from build123d import *

# Parameters (mm, degrees)
SKETCH_1_R          = 2.3
EXTRUDE_1_DEPTH     = 12
SKETCH_2_R          = 5.05
CUT_EXTRUDE_1_DEPTH = 3
CUT_EXTRUDE_START   = -3
SKETCH_3_R          = 5.05
CUT_EXTRUDE_2_DEPTH = 3
SKETCH_4_R          = 4
CUT_EXTRUDE_3_DEPTH = 15
CUT_EXTRUDE_4_DEPTH = 15
CHAMFER_1_SIZE      = 3
EXTRUDE_2_DEPTH     = 12
SKETCH_8_R          = 3
CUT_EXTRUDE_5_DEPTH = 12
CHAMFER_2_SIZE      = 3
SKETCH_9_R          = 2.3
EXTRUDE_4_DEPTH     = 4
FILLET_1_R          = 0.5
CUT_EXTRUDE_6_DEPTH = 22
SKETCH_11_R         = 4.05
CUT_EXTRUDE_7_DEPTH = 3
FILLET_2_R          = 0.5


with BuildPart() as part:
    # 草图1 → 凸台-拉伸1 (new body)
    with BuildSketch(Plane.XY):
        Polygon((-3.615367776, 90), (-7.5, -40), (-7.5, -80), (7.5, -80), (7.5, -40), (3.615367776, 90), align=None)
        with Locations((0, -74)):
            Circle(SKETCH_1_R, mode=Mode.SUBTRACT)
    extrude(amount=EXTRUDE_1_DEPTH)

    # 草图2 → 切除-拉伸1 (cut)
    with BuildSketch(Plane.XY.offset(12)):
        with Locations((0, -45)):
            Circle(SKETCH_2_R)
    extrude(amount=-CUT_EXTRUDE_1_DEPTH, mode=Mode.SUBTRACT)

    # 草图3 → 切除-拉伸2 (cut)
    with BuildSketch(Plane(origin=(0, 0, 0), x_dir=(-1, 0, 0), z_dir=(0, 0, -1)).offset(CUT_EXTRUDE_START)):
        with Locations(Location((0, -45, 0), (0, 0, 180))):
            Circle(SKETCH_3_R)
    extrude(amount=CUT_EXTRUDE_2_DEPTH, mode=Mode.SUBTRACT)

    # 草图4 → 切除-拉伸3 (cut)
    with BuildSketch(Plane.XY.offset(9)):
        with Locations((0, -45)):
            Circle(SKETCH_4_R)
    extrude(amount=-CUT_EXTRUDE_3_DEPTH, mode=Mode.SUBTRACT)

    # 草图6 → 切除-拉伸4 (cut)
    with BuildSketch(Plane.XY.offset(12)):
        Polygon((4.888073513, -27.298220102), (4.403458128, -9.298220102), (-4.403458128, -9.298220102), (-4.888073513, -27.298220102), align=None)
        Polygon((-3.86499659, 10.701779898), (3.86499659, 10.701779898), (4.349611974, -7.298220102), (-4.349611974, -7.298220102), align=None)
        Polygon((-2.734227359, 52.701779898), (2.734227359, 52.701779898), (2.249611974, 70.701779898), (-2.249611974, 70.701779898), align=None)
        Polygon((-3.272688897, 32.701779898), (3.272688897, 32.701779898), (2.788073513, 50.701779898), (-2.788073513, 50.701779898), align=None)
        Polygon((-3.811150436, 12.701779898), (3.811150436, 12.701779898), (3.326535051, 30.701779898), (-3.326535051, 30.701779898), align=None)
    extrude(amount=-CUT_EXTRUDE_4_DEPTH, mode=Mode.SUBTRACT)

    # 倒角1
    chamfer_1_edges = [part.edges().sort_by_distance(p)[0] for p in [
        (7.5, -80, 6),
        (-7.5, -80, 6),
    ]]
    chamfer(chamfer_1_edges, length=CHAMFER_1_SIZE)

    # 草图7 → 凸台-拉伸2 (add)
    with BuildSketch(Plane.XY.offset(12)):
        Polygon((-3.844369998, 82.33639451), (3.844369998, 82.33639451), (8.779475305, 87.271499817), (8.779475305, 96.223058652), (-8.779475305, 96.223058652), (-8.779475305, 87.271499817), align=None)
    extrude(amount=-EXTRUDE_2_DEPTH)

    # 草图8 → 切除-拉伸5 (cut)
    with BuildSketch(Plane.XY.offset(12)):
        with Locations((0, 89)):
            Circle(SKETCH_8_R)
    extrude(amount=-CUT_EXTRUDE_5_DEPTH, mode=Mode.SUBTRACT)

    # 倒角2
    chamfer_2_edges = [part.edges().sort_by_distance(p)[0] for p in [
        (-8.779475305, 96.223058652, 6),
        (8.779475305, 96.223058652, 6),
    ]]
    chamfer(chamfer_2_edges, length=CHAMFER_2_SIZE)

    # 草图9 → 凸台-拉伸4 (add)
    with BuildSketch(Plane.XY.offset(12)):
        Polygon((-7.5, -70), (-4.5, -65), (4.5, -65), (7.5, -70), (7.5, -77), (4.5, -80), (-4.5, -80), (-7.5, -77), align=None)
        with Locations((0, -74)):
            Circle(SKETCH_9_R, mode=Mode.SUBTRACT)
    extrude(amount=EXTRUDE_4_DEPTH)

    # 圆角1
    fillet_1_edges = [part.edges().sort_by_distance(p)[0] for p in [
        (-5.05, -45, 12),
        (-5.05, -45, 0),
    ]]
    fillet(fillet_1_edges, radius=FILLET_1_R)

    # 草图10 → 切除-拉伸6 (cut)
    with BuildSketch(Plane.XY.offset(12)):
        with BuildLine():
            Line((-5.779475305, 96.223058652), (0, 96.223058652))
            ThreePointArc((0, 96.223058652), (-6.94052162, 91.000433937), (-3.844369998, 82.884986049))
            Line((-3.844369998, 82.884986049), (-3.844369998, 82.33639451))
            Line((-3.844369998, 82.33639451), (-8.779475305, 87.271499817))
            Line((-8.779475305, 87.271499817), (-8.779475305, 93.223058652))
            Line((-8.779475305, 93.223058652), (-5.779475305, 96.223058652))
        make_face()
    extrude(amount=-CUT_EXTRUDE_6_DEPTH, mode=Mode.SUBTRACT)

    # 草图11 → 切除-拉伸7 (cut)
    with BuildSketch(Plane.XY.offset(12)):
        with Locations((0, 89)):
            Circle(SKETCH_11_R)
    cut_extrude_7 = extrude(amount=-CUT_EXTRUDE_7_DEPTH, mode=Mode.SUBTRACT)

    # 镜向1: 切除-拉伸7 across plane
    add(cut_extrude_7.mirror(Plane.XY.offset(6)), mode=Mode.SUBTRACT)

    # 圆角2
    fillet_2_edges = [part.edges().sort_by_distance(p)[0] for p in [
        (-4.05, 89, 12),
        (-4.05, 89, 0),
    ]]
    fillet(fillet_2_edges, radius=FILLET_2_R)


solid = part.part
The model under review builds one solid part; all positions refer to its coordinate system, in mm. A direction names the side the tool comes from. Round coordinates to 2 decimals unless told otherwise and drop trailing zeros. Loops run counter-clockwise (first coordinate to the right, second up) from the corner with the lowest first, then second, coordinate; pieces in that order, holes last. Notation, with made-up numbers: M 32,79 L 50,79 A14 ccw 50,93 Z; hole C -4,-3.5 d11. An arc over 180 degrees is marked long. Answer as CSV lines item,"result". Start each with the question number.
Item 1: Consider section A-A (y = -45). Write out the cut boundary in (x, z), then the cut area to 3 significant figures.
Item 2: Consider section D-D (y = -74). Write out the cut boundary in (x, z), then the cut area to 3 significant figures.
Item 3: Insertion check: P1, Ø5, axis at x = 1.5, y = -44, coming from the -Z side; P2, Ø6, axis at y = 39, z = 5, coming from the -X side; P3, Ø4, axis at y = 63.5, z = 5, coming from the +X side; P4, Ø4.5, axis at x = -1, z = 13, coming from the +Y side. Each pin has a flat end and moves straight along its axis. Give the tip position at first contact, or say it passes through.
Item 4: Consider section C-C (y = 89). Write out the cut boundary in (x, z), then the cut area to 3 significant figures.
Item 5: Consider section B-B (z = 7). State how many separate pieces and enclosed holes the cut face has, then the cut area to 3 significant figures.
Item 6: Mouldability with a two-part tool opening along Y and no side actions: class faces 5 (the face through (0, -80, 8)), 6 (the face through (8.779, 90, 6)), 7 (the face through (0, 52.702, 6)) as released by +Y, released by -Y, zero draft, split by the parting line, or undercut.
Item 7: Wall thickness on line 1 (Z direction, x = -1.75, y = 31); line 2 (X direction, y = -11, z = 5.5); line 3 (X direction, y = 44.5, z = 9.75): over which ranges is each line inside the solid? List them lowest first. Write a range as [from, to].
Item 8: For faces 1 (the face through (6, -67.5, 14)), 2 (the face through (2.33, -40.52, 1.77)), 3 (the face through (7.5, -59, 6)), 4 (the face through (0, 12.702, 6)), list the 3-axis set-ups (+Z, -Z, +X, -X, +Y, -Y) from which the entire face can be reached by the end or side of a thin tool; tool diameter is ignored.
Answer:
1,outline,"M -7.5,0 L -5.55,0 A0.5 ccw -5.05,0.5 L -5.05,3 L -4,3 L -4,9 L -5.05,9 L -5.05,11.5 A0.5 ccw -5.55,12 L -7.5,12 Z; M 4,3 L 5.05,3 L 5.05,0.5 A0.5 ccw 5.55,0 L 7.5,0 L 7.5,12 L 5.55,12 A0.5 ccw 5.05,11.5 L 5.05,9 L 4,9 Z"
1,area,"71.2 mm^2"
2,outline,"M -7.5,0 L -2.3,0 L -2.3,16 L -7.5,16 Z; M 2.3,0 L 7.5,0 L 7.5,16 L 2.3,16 Z"
2,area,"166 mm^2"
3,P1,"stops at z = 3"
3,P2,"stops at x = -5.23"
3,P3,"stops at x = 4.47"
3,P4,"stops at y = 96.22"
4,outline,"M -7.22,0 L -4.55,0 A0.5 ccw -4.05,0.5 L -4.05,3 L -3,3 L -3,9 L -4.05,9 L -4.05,11.5 A0.5 ccw -4.55,12 L -7.22,12 Z; M 3,3 L 4.05,3 L 4.05,0.5 A0.5 ccw 4.55,0 L 8.78,0 L 8.78,12 L 4.55,12 A0.5 ccw 4.05,11.5 L 4.05,9 L 3,9 Z"
4,area,"107 mm^2"
5,separate pieces,"1"
5,enclosed holes,"8"
5,area,"1,430 mm^2"
6,face 5,"released by -Y"
6,face 6,"zero draft"
6,face 7,"undercut"
7,line 1,"z = [0, 12]"
7,line 2,"x = [-6.63, -4.45], [4.45, 6.63]"
7,line 3,"x = [-4.97, -2.96], [2.96, 4.97]"
8,face 1,"+Z, +X, +Y"
8,face 2,"-Z"
8,face 3,"+Z, -Z, +X, -Y"
8,face 4,"+Z, -Z"
